from build123d import *

# Parameters (mm, degrees)
SKETCH1_W           = 9.525
SKETCH1_H           = 48.26
SKETCH1_R           = 3.302
BOSS_EXTRUDE1_DEPTH = 9.525
FILLET1_R           = 5.08


with BuildPart() as part:
    # Sketch1 → Boss-Extrude1 (new body)
    with BuildSketch(Plane.XY):
        Rectangle(SKETCH1_W, SKETCH1_H)
        with Locations(Location((0, -17.78, 0), (0, 0, 180))):
            Circle(SKETCH1_R, mode=Mode.SUBTRACT)
        with Locations(Location((0, 17.78, 0), (0, 0, 180))):
            Circle(SKETCH1_R, mode=Mode.SUBTRACT)
    extrude(amount=BOSS_EXTRUDE1_DEPTH)

    # Fillet1
    # the kernel refuses this fillet: 5.08 mm, written as the material it takes off along each edge
    with BuildSketch(Plane(origin=(-4.7625, -24.13, -12.7), x_dir=(1, 0, 0), z_dir=(0, 0, 1)), Plane(origin=(4.7625, -24.13, -12.7), x_dir=(0, 1, 0), z_dir=(0, 0, 1)), Plane(origin=(4.7625, 24.13, -12.7), x_dir=(-1, 0, 0), z_dir=(0, 0, 1))) as fillet1_piece_1:
        with BuildLine():
            CenterArc((FILLET1_R, FILLET1_R), FILLET1_R, 180, 90)
            Line((0, FILLET1_R), (0, 0))
            Line((0, 0), (FILLET1_R, 0))
        make_face()
    extrude(amount=34.925, mode=Mode.SUBTRACT)
    with BuildSketch(Plane(origin=(-4.7625, 24.13, -12.7), x_dir=(1, 0, 0), z_dir=(0, 0, 1))) as fillet1_piece_2:
        with BuildLine():
            CenterArc((FILLET1_R, -FILLET1_R), FILLET1_R, 90, 90)
            Line((0, -FILLET1_R), (0, 0))
            Line((0, 0), (FILLET1_R, 0))
        make_face()
    extrude(amount=34.925, mode=Mode.SUBTRACT)


solid = part.part
The listing builds one solid part. Answer for the finished solid, in the listing's coordinates (mm). Coordinates: 2 decimals unless noted, no trailing zeros. Write each loop counter-clockwise with the first axis right and the second up, starting at its lowest first coordinate (ties: lowest second). Pieces come first, ordered by that corner, then holes. Notation, with made-up numbers: M 14,15 L 32,15 A4 cw 32,20 Z; hole C 32.25,71 d4. An arc over 180 degrees is marked long. Write each question's results on one line, items separated by ' | '.
Item 1: The part is cut by section D-D on y = -15.5. Determine the outline of the cut face in (x, z) (1 decimal), and give its area (3 significant figures).
Answer below:
outline: M -4.8,0 L -2.4,0 L -2.4,9.5 L -4.8,9.5 Z; M 2.4,0 L 4.8,0 L 4.8,9.5 L 2.4,9.5 Z | area: 45.2 mm2
Item 2: The part is cut by section B-B on z = 5.75. Determine the outline of the cut face in (x, y).
Answer below:
outline: M -4.76,-19.05 A5.08 ccw 0,-24.12 A5.08 ccw 4.76,-19.05 L 4.76,19.05 A5.08 ccw 0,24.12 A5.08 ccw -4.76,19.05 Z; hole C 0,-17.78 d6.6; hole C 0,17.78 d6.6
Item 3: The part is cut by section C-C on x = -2.5. Determine the outline of the cut face in (y, z) (3 decimals), and give its area (3 significant figures).
Answer below:
outline: M -23.277,0 L -19.937,0 L -19.937,9.525 L -23.277,9.525 Z; M -15.623,0 L 15.623,0 L 15.623,9.525 L -15.623,9.525 Z; M 19.937,0 L 23.277,0 L 23.277,9.525 L 19.937,9.525 Z | area: 361 mm2
Item 4: The part is cut by section A-A on y = 17.78. Determine the outline of the cut face in (x, z) (1 decimal).
Answer below:
outline: M -4.8,0 L -3.3,0 L -3.3,9.5 L -4.8,9.5 Z; M 3.3,0 L 4.8,0 L 4.8,9.5 L 3.3,9.5 Z
Item 5: Consider probe 1 along Y at (x, z) = (0.75, 4.75); probe 2 along X at (y, z) = (-18, 6.75); probe 3 along Y at (x, z) = (-2.25, 2.25). Determine where each line is inside the solid, lowest interval first. Write a range as [from, to].
Answer below:
probe 1: [-24.02, -21], [-14.56, 14.56], [21, 24.02] | probe 2: [-4.76, -3.29], [3.29, 4.76] | probe 3: [-23.43, -20.2], [-15.36, 15.36], [20.2, 23.43]
Item 6: Given P1, Ø2, axis at x = -2.5, z = 5, coming from the +Y side; P2, Ø1, axis at x = -2.5, z = 1.5, coming from the -Y side; P3, Ø3, axis at x = -3, z = 3.5, coming from the -Y side; P4, Ø1, axis at x = 2, y = 18.5, coming from the -Z side, each flat-ended and moving along its own axis, determine where each tip first touches the part or whether it passes through.
Answer below:
P1: y = 23.79 | P2: y = -23.57 | P3: y = -23.79 | P4: through
Item 7: For a pull along Y with two mould halves and no side action, classify faces 1 (the face through (-1.52, 20.71, 4.7)), 2 (the face through (-3.348, 22.567, 4.696)), 3 (the face through (-4.762, 0, 5)) as released by +Y, released by -Y, zero draft, split by the parting line, or undercut.
Answer below:
face 1: undercut | face 2: released by +Y | face 3: zero draft
